```python
from build123d import *

# Parameters (mm, degrees)
ESQUISSE1_R        = 2.5
ESQUISSE1_W        = 25
ESQUISSE1_H        = 7.609144865
BOSS_EXTRU_1_DEPTH = 9
ESQUISSE2_W        = 49.997440748
ESQUISSE2_H        = 8
BOSS_EXTRU_2_DEPTH = 50


with BuildPart() as part:
    # Esquisse1 → Boss.-Extru.1 (new body)
    with BuildSketch(Plane.XY):
        Polygon((1.553236782, 0), (81.553236782, 0), (81.553236782, 8), (66.553236782, 8), (66.553236782, 83), (16.553236782, 83), (16.553236782, 8), (1.553236782, 8), align=None)
        with Locations((41.553236782, 46.5)):
            Circle(ESQUISSE1_R, mode=Mode.SUBTRACT)
        with Locations((41.553236782, 66.5)):
            Circle(ESQUISSE1_R, mode=Mode.SUBTRACT)
        with Locations((41.553236782, 56.667811129)):
            Rectangle(ESQUISSE1_W, ESQUISSE1_H, mode=Mode.SUBTRACT)
    extrude(amount=-BOSS_EXTRU_1_DEPTH)

    # Esquisse2 → Boss.-Extru.2 (add)
    with BuildSketch(Plane.XY):
        with Locations((41.551957156, 4)):
            Rectangle(ESQUISSE2_W, ESQUISSE2_H)
    extrude(amount=BOSS_EXTRU_2_DEPTH)


solid = part.part
```
The listing builds one solid part. Answer for the finished solid, in the listing's coordinates (mm). A direction names the side the tool comes from. Coordinates: 2 decimals unless noted, no trailing zeros. Write each loop counter-clockwise with the first axis right and the second up, starting at its lowest first coordinate (ties: lowest second). Pieces come first, ordered by that corner, then holes. Notation, with made-up numbers: (-34.75, 20) - (-2.75, 20) arc R26 ccw to (-2.75, 50) - close; hole circle Ø6 at (60.25, -39.5). An arc over 180 degrees is marked (long way). One line per item, written item: value.
1) Find section B-B (y = 66.5). Give the vertices of the cut face in (x, z), and give its area (3 significant figures).
Geometry check:
outline: (16.55, -9) - (39.05, -9) - (39.05, 0) - (16.55, 0) - close; (44.05, -9) - (66.55, -9) - (66.55, 0) - (44.05, 0) - close
area: 405 mm2
2) Find section A-A (x = 45.5). Give the vertices of the cut face in (y, z).
Geometry check:
outline: (0, -9) - (52.86, -9) - (52.86, 0) - (8, 0) - (8, 50) - (0, 50) - close; (60.47, -9) - (83, -9) - (83, 0) - (60.47, 0) - close
3) Consider line 1 along Z through (x, y) = (26, 71); line 2 along Y through (x, z) = (62, 22). Determine where each line is inside the solid, lowest interval first. Write a range as from..to.
Geometry check:
line 1: z = -9..0
line 2: y = 0..8
4) Each of these flat-tipped pins is pushed along its axis until it touches: pin 1 Ø8.5 at (y, z) = (57.5, -4) entering from -X; pin 2 Ø7 at (x, z) = (7, -2.5) entering from +Y; pin 3 Ø8 at (x, y) = (46.5, 53.5) entering from +Z. Where does it stop, or does it pass through?
Geometry check:
pin 1: stops at x = 16.55
pin 2: stops at y = 8
pin 3: stops at z = 0
5) Find section D-D (y = 55.5). Give the vertices of the cut face in (x, z), and give its area (3 significant figures).
Geometry check:
outline: (16.55, -9) - (29.05, -9) - (29.05, 0) - (16.55, 0) - close; (54.05, -9) - (66.55, -9) - (66.55, 0) - (54.05, 0) - close
area: 225 mm2
6) A tool of negligible diameter and unlimited length cuts with its end or side. For faces 1 (the flat face through (9, 8, -4)), 2 (the flat face through (29.053, 57, -4)), 3 (the flat face through (66.551, 4, 25)), from which of +Z, -Z, +X, -X, +Y, -Y can it reach the whole face along a straight path? Write none if from no direction.
Geometry check:
face 1: +Z, -Z, -X, +Y
face 2: +Z, -Z
face 3: +Z, +X, +Y, -Y
7) Find section C-C (z = -4.5). Give the vertices of the cut face in (x, y).
Geometry check:
outline: (1.55, 0) - (81.55, 0) - (81.55, 8) - (66.55, 8) - (66.55, 83) - (16.55, 83) - (16.55, 8) - (1.55, 8) - close; hole (29.05, 52.86) - (54.05, 52.86) - (54.05, 60.47) - (29.05, 60.47) - close; hole circle Ø5 at (41.55, 46.5); hole circle Ø5 at (41.55, 66.5)
8) For a pull along X with two mould halves and no side action, classify faces 4 (the flat face through (16.553, 46, -4)), 5 (the cylindrical face through (43.86, 45.54, -4.44)), 6 (the flat face through (41, 60.472, -4)), 7 (the flat face through (66.553, 45, -4)) as pulls with the +X half, pulls with the -X half, needs draft (parallel to the pull), parting line crosses it, or undercut.
Geometry check:
face 4: pulls with the -X half
face 5: undercut
face 6: undercut
face 7: pulls with the +X half
